Geometry check sheet. Reference: the model listing, model coordinates, mm. Give positions to 0.01 mm unless a question says otherwise; leave off trailing zeros. Write each loop counter-clockwise with the first axis right and the second up, starting at its lowest first coordinate (ties: lowest second). Pieces come first, ordered by that corner, then holes. Notation, with made-up numbers: M 26.25,76.5 L 59.25,76.5 A20 ccw 59.25,112.5 Z; hole C -7.75,73.5 d3. An arc over 180 degrees is marked long. Write each question's results on one line, items separated by ' | '.
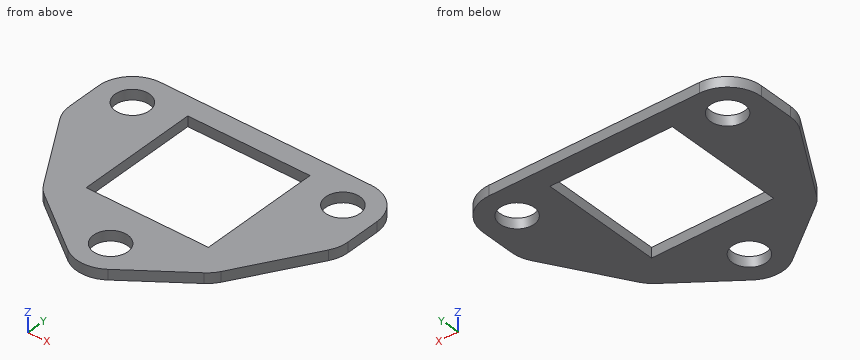
Autodesk Inventor part; units mm, degrees
ref_plane "YZ Plane" through (0, 0, 0) normal (1, 0, 0) x (0, 1, 0)
ref_plane "XZ Plane" through (0, 0, 0) normal (0, 1, 0) x (-1, 0, 0)
ref_plane "XY Plane" through (0, 0, 0) normal (0, 0, 1) x (1, 0, 0)
sketch "Sketch6" plane through (0, 0, 0) normal (0, 0, 1) x (1, 0, 0)
  line L0 (18, 18) -> (-18, 18)
  line L1 (-18, 18) -> (-18, -18)
  line L2 (-18, -18) -> (18, -18)
  line L3 (18, -18) -> (18, 18)
  line L4 (18, 18) -> (-18, -18) construction
  circle A0 centre (0, -31) radius 5.05
  circle A1 centre (31, 14) radius 5.05
  circle A2 centre (-31, 14) radius 5.05
  line L5 (31, 14) -> (-31, 14) construction
  line L6 (-31, 14) -> (0, -31) construction
  line L7 (0, -31) -> (31, 14) construction
  line L8 (0, 18) -> (0, -18) construction
  line L9 (-41, 24) -> (41, 24)
  line L10 (41, 24) -> (41, 1)
  line L11 (41, 1) -> (25.1414, -25)
  line L12 (25.1414, -25) -> (0, -43.3896)
  line L13 (-41, 24) -> (-41, 1)
  line L14 (-41, 1) -> (-25.1414, -25)
  line L15 (-25.1414, -25) -> (0, -43.3896)
  point P0 (0, 0)
  point P1 (0, 0)
  point P2 (60, 0)
  dimension "d30" = 36
  dimension "d31" = 36
  dimension "d33" = 10.1
  dimension "d37" = 54.6443
  dimension "d43" = 13
  dimension "d44" = 13
  dimension "d45" = 6
  dimension "d46" = 10
  dimension "d47" = 10
  dimension "d48" = 10
  dimension "d49" = 23
  dimension "d50" = 7
  dimension "d51" = 10
extrude "Plate3" add sketch "Sketch6" along normal blind 3
fillet "Corner Round1" radius 10 7 edges at (-41, 24, 1.5) (41, 24, 1.5) (41, 1, 1.5) (25.1414, -25, 1.5) (0, -43.3896, 1.5) (-25.1414, -25, 1.5) (-41, 1, 1.5)
equation "\"d41\" = Thickness"
equation "\"BendReliefWidth\" = Thickness"
equation "\"BendReliefDepth\" = 0.5 * Thickness"
equation "\"CornerReliefSize\" = 4 * Thickness"
equation "\"MinimumRemnant\" = 2 * Thickness"
equation "\"TransitionRadius\" = BendRadius"
equation "\"JacobiRadiusSize\" = BendRadius"
equation "\"GapSize\" = Thickness"
properties part number "MNT-CDF-504 small tube flange" material "Stainless Steel"
Q1. Section check B-B (y = -34). Enter the section's corners in (x, z).
Answer key:
outline: M -12.84,0 L -4.06,0 L -4.06,3 L -12.84,3 Z; M 4.06,0 L 12.84,0 L 12.84,3 L 4.06,3 Z
Q2. Depth check by flat-ended pin: P1, Ø1, axis at y = -17, z = 0.5, coming from the -X side. Enter the tip coordinate at first touch or a pass-through.
Answer key:
P1: stops at x = -30.33
Q3. Section check C-C (z = 2.35). Enter the section's corners in (x, y).
Answer key:
outline: M -41,3.81 A10 ccw -39.54,-1.4 L -26.17,-23.31 A10 ccw -23.54,-26.17 L -5.9,-39.07 A10 ccw 5.9,-39.07 L 23.54,-26.17 A10 ccw 26.17,-23.31 L 39.54,-1.4 A10 ccw 41,3.81 L 41,14 A10 ccw 31,24 L -31,24 A10 ccw -41,14 Z; hole C -31,14 d10.1; hole M -18,-18 L 18,-18 L 18,18 L -18,18 Z; hole C 0,-31 d10.1; hole C 31,14 d10.1
Q4. Section check A-A (x = 0). Enter the section's corners in (y, z), then the cut area to 3 significant figures.
Answer key:
outline: M -41,0 L -36.05,0 L -36.05,3 L -41,3 Z; M -25.95,0 L -18,0 L -18,3 L -25.95,3 Z; M 18,0 L 24,0 L 24,3 L 18,3 Z | area: 56.7 mm2
Q5. Material ranges on probe 1 along Y at (x, z) = (0, 0.7); probe 2 along X at (y, z) = (6.5, 2); probe 3 along X at (y, z) = (12, 0.7), recorded low to high. Write a range as [from, to].
Answer key:
probe 1: y = [-41, -36.05], [-25.95, -18], [18, 24] | probe 2: x = [-41, -18], [18, 41] | probe 3: x = [-41, -35.64], [-26.36, -18], [18, 26.36], [35.64, 41]
Q6. Section check D-D (x = 13). Enter the section's corners in (y, z), then the cut area to 3 significant figures.
Answer key:
outline: M -33.88,0 L -18,0 L -18,3 L -33.88,3 Z; M 18,0 L 24,0 L 24,3 L 18,3 Z | area: 65.6 mm2
